from build123d import *

# Parameters (mm, degrees)
SKETCH1_W                = 25.5
SKETCH1_H                = 25.5
BOSS_EXTRUDE1_DEPTH      = 25.5
SKETCH2_W                = 23.1
SKETCH2_H                = 23.1
SKETCH2_W_2              = 20
SKETCH2_H_2              = 20
BOSS_EXTRUDE2_DEPTH      = 25.5
SKETCH3_W                = 23.1
SKETCH3_H                = 23.1
SKETCH3_W_2              = 20
SKETCH3_H_2              = 20
BOSS_EXTRUDE3_DEPTH      = 25.5
SKETCH4_W                = 23.1
SKETCH4_H                = 23.1
SKETCH4_W_2              = 20
SKETCH4_H_2              = 20
BOSS_EXTRUDE4_DEPTH      = 25.5
FILLET4_R                = 1
F_6_0_6_DIAMETER_HOLE1_D = 6
F_6_0_6_DIAMETER_HOLE2_D = 6


with BuildPart() as part:
    # Sketch1 → Boss-Extrude1 (new body)
    with BuildSketch(Plane.XY):
        Rectangle(SKETCH1_W, SKETCH1_H)
    extrude(amount=BOSS_EXTRUDE1_DEPTH)

    # Sketch2 → Boss-Extrude2 (add)
    with BuildSketch(Plane(origin=(0, 12.75, 0), x_dir=(1, 0, 0), z_dir=(0, 1, 0))):
        with Locations((0, -12.75)):
            Rectangle(SKETCH2_W, SKETCH2_H)
        with Locations((0, -12.75)):
            Rectangle(SKETCH2_W_2, SKETCH2_H_2, mode=Mode.SUBTRACT)
    extrude(amount=BOSS_EXTRUDE2_DEPTH)

    # Sketch3 → Boss-Extrude3 (add)
    with BuildSketch(Plane.XY.offset(25.5)):
        Rectangle(SKETCH3_W, SKETCH3_H)
        Rectangle(SKETCH3_W_2, SKETCH3_H_2, mode=Mode.SUBTRACT)
    extrude(amount=BOSS_EXTRUDE3_DEPTH)

    # Sketch4 → Boss-Extrude4 (add)
    with BuildSketch(Plane.ZY.offset(12.75)):
        with Locations((12.75, 0)):
            Rectangle(SKETCH4_W, SKETCH4_H)
        with Locations((12.75, 0)):
            Rectangle(SKETCH4_W_2, SKETCH4_H_2, mode=Mode.SUBTRACT)
    extrude(amount=BOSS_EXTRUDE4_DEPTH)

    # Fillet4
    fillet4_edges = [part.edges().sort_by_distance(p)[0] for p in [
        (11.55, 38.25, 12.75),
        (0, 38.25, 1.2),
        (-11.55, 38.25, 12.75),
        (0, 38.25, 24.3),
        (11.55, 25.5, 24.3),
        (11.55, 25.5, 1.2),
        (-11.55, 25.5, 1.2),
        (-11.55, 25.5, 24.3),
        (11.55, 0, 51),
        (0, 11.55, 51),
        (-11.55, 0, 51),
        (0, -11.55, 51),
        (11.55, -11.55, 38.25),
        (11.55, 11.55, 38.25),
        (-11.55, 11.55, 38.25),
        (-11.55, -11.55, 38.25),
        (-38.25, 0, 24.3),
        (-38.25, 11.55, 12.75),
        (-38.25, 0, 1.2),
        (-38.25, -11.55, 12.75),
        (-25.5, -11.55, 24.3),
        (-25.5, 11.55, 24.3),
        (-25.5, 11.55, 1.2),
        (-25.5, -11.55, 1.2),
    ]]
    fillet(fillet4_edges, radius=FILLET4_R)

    # Ø6.0 (6) Diameter Hole1 (through all)
    with Locations(Plane(origin=(0, 0, 1.2), x_dir=(-1, 0, 0), z_dir=(0, 0, -1))):
        with Locations((24.55, -0.15)):
            Hole(F_6_0_6_DIAMETER_HOLE1_D / 2)

    # Ø6.0 (6) Diameter Hole2 (through all)
    with Locations(Plane(origin=(11.55, 0, 0), x_dir=(0, 0, -1), z_dir=(1, 0, 0))):
        with Locations((-37.3, -0.15)):
            Hole(F_6_0_6_DIAMETER_HOLE2_D / 2)


solid = part.part
Model file for the job. Use its own axes, mm. A direction names the side the tool comes from. Round coordinates to 2 decimals unless told otherwise and drop trailing zeros. Loops run counter-clockwise (first coordinate to the right, second up) from the corner with the lowest first, then second, coordinate; pieces in that order, holes last. Notation, with made-up numbers: (-27.75, -19) -> (-20.75, -19) arc R22 ccw to (-20.75, 20) -> close; hole circle Ø2 at (70.25, -2). An arc over 180 degrees is marked (long way). Answer as CSV lines item,"result". Start each with the question number.
1) Tool access for faces 1 (the face through (-12.75, -0.1, 0.4)), 2 (the face through (10, 0, 41)), 3 (the face through (0, 12.75, 13)), 4 (the face through (-25, -11.55, 13)): list every direction of +Z, -Z, +X, -X, +Y, -Y with a clear straight run to the whole face (end or side of a thin tool).
2) Slice it at B-B (z = 37.3). List the corners of the cut face in (x, y).
3) Mould opens along Z. For faces 5 (the face through (0, 25, 1.2)), 6 (the face through (-10.2, 0, 51)), 7 (the face through (-28, 0, 22.75)), 8 (the face through (-11.55, 2, 40)) say: +Z half, -Z half, draft (parallel to the pull), parting line (faces both ways), or undercut.
4) Probe line 1 along Y through (x, z) = (10.7, 37.3); line 2 along X through (y, z) = (-0.5, 31.5). List the from-to ranges inside material, lowest first.
5) Pin check, flat tips, straight feed: P1, Ø10.5, axis at y = 30.5, z = 12.5, coming from the -X side; P2, Ø1, axis at x = -18, z = 24, coming from the +Y side; P3, Ø3, axis at x = -13.5, z = 42.5, coming from the -Y side; P4, Ø3, axis at x = -15.5, z = 13, coming from the -Y side. Stop position of each tip, or through.
6) Slice it at D-D (y = 9). List the corners of the cut face in (x, z).
7) Slice it at C-C (y = 32). List the corners of the cut face in (x, z), plus the area to 3 significant figures.
8) Slice it at A-A (x = -24.55). List the corners of the cut face in (y, z).
Filled in:
1,face 1,"-X"
1,face 2,"+Z"
1,face 3,"+Y"
1,face 4,"+Z, -Z, -X, -Y"
2,outline,"(-11.55, -10.55) arc R1 ccw to (-10.55, -11.55) -> (10.55, -11.55) arc R1 ccw to (11.55, -10.55) -> (11.55, -3.15) -> (10, -3.15) -> (10, -10) -> (-10, -10) -> (-10, -3.15) -> (-11.55, -3.15) -> close; (-11.55, 2.85) -> (-10, 2.85) -> (-10, 10) -> (10, 10) -> (10, 2.85) -> (11.55, 2.85) -> (11.55, 10.55) arc R1 ccw to (10.55, 11.55) -> (-10.55, 11.55) arc R1 ccw to (-11.55, 10.55) -> close"
3,face 5,"-Z half"
3,face 6,"+Z half"
3,face 7,"undercut"
3,face 8,"draft"
4,line 1,"y = -11.54 to -3.15, 2.85 to 11.54"
4,line 2,"x = -11.55 to -10, 10 to 11.55"
5,P1,"stops at x = -11.55"
5,P2,"stops at y = 11.53"
5,P3,"passes through"
5,P4,"stops at y = -11.55"
6,outline,"(-38.25, 2.2) arc R1 ccw to (-37.25, 1.2) -> (-12.75, 1.2) -> (-12.75, 0) -> (12.75, 0) -> (12.75, 25.5) -> (11.55, 25.5) -> (11.55, 50) arc R1 ccw to (10.55, 51) -> (10, 51) -> (10, 25.5) -> (-10, 25.5) -> (-10, 51) -> (-10.55, 51) arc R1 ccw to (-11.55, 50) -> (-11.55, 25.5) -> (-12.75, 25.5) -> (-12.75, 24.3) -> (-37.25, 24.3) arc R1 ccw to (-38.25, 23.3) -> (-38.25, 22.75) -> (-12.75, 22.75) -> (-12.75, 2.75) -> (-38.25, 2.75) -> close"
7,outline,"(-11.55, 2.2) arc R1 ccw to (-10.55, 1.2) -> (10.55, 1.2) arc R1 ccw to (11.55, 2.2) -> (11.55, 23.3) arc R1 ccw to (10.55, 24.3) -> (-10.55, 24.3) arc R1 ccw to (-11.55, 23.3) -> close; hole (-10, 2.75) -> (10, 2.75) -> (10, 22.75) -> (-10, 22.75) -> close"
7,area,"133 mm2"
8,outline,"(-11.55, 2.2) arc R1 ccw to (-10.55, 1.2) -> (-3.15, 1.2) -> (-3.15, 2.75) -> (-10, 2.75) -> (-10, 22.75) -> (-3.15, 22.75) -> (-3.15, 24.3) -> (-10.55, 24.3) arc R1 ccw to (-11.55, 23.3) -> close; (2.85, 1.2) -> (10.55, 1.2) arc R1 ccw to (11.55, 2.2) -> (11.55, 23.3) arc R1 ccw to (10.55, 24.3) -> (2.85, 24.3) -> (2.85, 22.75) -> (10, 22.75) -> (10, 2.75) -> (2.85, 2.75) -> close"
